from build123d import *

# Parameters (mm, degrees)
SKETCH1_R           = 13.49375
BOSS_EXTRUDE1_DEPTH = 2.54
CUT_EXTRUDE1_START  = -3.54
SKETCH2_R           = 1.5875
CUT_EXTRUDE1_DEPTH  = 4.54
CIRPATTERN1_COUNT   = 12


with BuildPart() as part:
    # Sketch1 → Boss-Extrude1 (new body)
    with BuildSketch(Plane(origin=(0, 0, 0), x_dir=(1, 0, 0), z_dir=(0, 1, 0))):
        Circle(SKETCH1_R)
    extrude(amount=BOSS_EXTRUDE1_DEPTH)

    # Sketch2 → Cut-Extrude1 (cut)
    with BuildSketch(Plane(origin=(0, 2.54, 0), x_dir=(1, 0, 0), z_dir=(0, 1, 0)).offset(CUT_EXTRUDE1_START)):
        with Locations((-9.525, 0)):
            Circle(SKETCH2_R)
    cut_extrude1 = extrude(amount=CUT_EXTRUDE1_DEPTH, mode=Mode.SUBTRACT)

    # CirPattern1: Cut-Extrude1 ×12 about axis
    cirpattern1_axis = Axis((0, 0, 0), (0, 1, 0))
    for i in range(1, CIRPATTERN1_COUNT):
        add(cut_extrude1.rotate(cirpattern1_axis, i * 360 / CIRPATTERN1_COUNT), mode=Mode.SUBTRACT)


solid = part.part
Check sheet for the modelled part. Datum: model origin and axes. Units: mm. Coordinates: 2 decimals unless noted, no trailing zeros. Write each loop counter-clockwise with the first axis right and the second up, starting at its lowest first coordinate (ties: lowest second). Pieces come first, ordered by that corner, then holes.
Item 1: Cross-section at D-D on x = 10.5. Record the boundary of the cut face in (y, z).
Numbers:
outline: (0, -8.48) - (2.54, -8.48) - (2.54, -1.25) - (0, -1.25) - close; (0, 1.25) - (2.54, 1.25) - (2.54, 8.48) - (0, 8.48) - close
Item 2: Scan lines: probe 1 along Z at (x, y) = (-8.25, 1.2) (3 decimals); probe 2 along Z at (x, y) = (-4.25, 2.2); probe 3 along X at (y, z) = (2.05, -3.5). Record each from-to range of solid material in increasing order.
Numbers:
probe 1: z = -10.678 to -6.35, -3.175 to -0.946, 0.946 to 3.175, 6.35 to 10.678
probe 2: z = -12.81 to -9.75, -6.75 to 6.75, 9.75 to 12.81
probe 3: x = -13.03 to -9.21, -7.29 to 7.29, 9.21 to 13.03
Item 3: Cross-section at C-C on z = -9.25. Record the boundary of the cut face in (x, y).
Numbers:
outline: (-9.82, 0) - (-5.99, 0) - (-5.99, 2.54) - (-9.82, 2.54) - close; (-3.53, 0) - (-1.56, 0) - (-1.56, 2.54) - (-3.53, 2.54) - close; (1.56, 0) - (3.53, 0) - (3.53, 2.54) - (1.56, 2.54) - close; (5.99, 0) - (9.82, 0) - (9.82, 2.54) - (5.99, 2.54) - close
Item 4: Mould release check, pull along X, two halves, no side actions. Record for faces 1 (the face through (6.277, 1.252, -8.726)), 2 (the face through (-9.945, 1.252, -9.12)), 3 (the face through (0, 0, 0)): released by +X, released by -X, zero draft, split by the parting line, or undercut.
Numbers:
face 1: undercut
face 2: split by the parting line
face 3: zero draft
Item 5: Cross-section at A-A on z = 0. Record the boundary of the cut face in (x, y), then the cut area to 3 significant figures.
Numbers:
outline: (-13.49, 0) - (-11.11, 0) - (-11.11, 2.54) - (-13.49, 2.54) - close; (-7.94, 0) - (7.94, 0) - (7.94, 2.54) - (-7.94, 2.54) - close; (11.11, 0) - (13.49, 0) - (13.49, 2.54) - (11.11, 2.54) - close
area: 52.4 mm2
Item 6: Depth check by flat-ended pin: pin 1 Ø3 at (x, z) = (4.76, -8.25) entering from -Y. Enter the tip coordinate at first touch or a pass-through.
Numbers:
pin 1: passes through
Item 7: Cross-section at B-B on x = 7.25. Record the boundary of the cut face in (y, z).
Numbers:
outline: (0, -11.38) - (2.54, -11.38) - (2.54, -6) - (0, -6) - close; (0, -3.53) - (2.54, -3.53) - (2.54, 3.53) - (0, 3.53) - close; (0, 6) - (2.54, 6) - (2.54, 11.38) - (0, 11.38) - close
